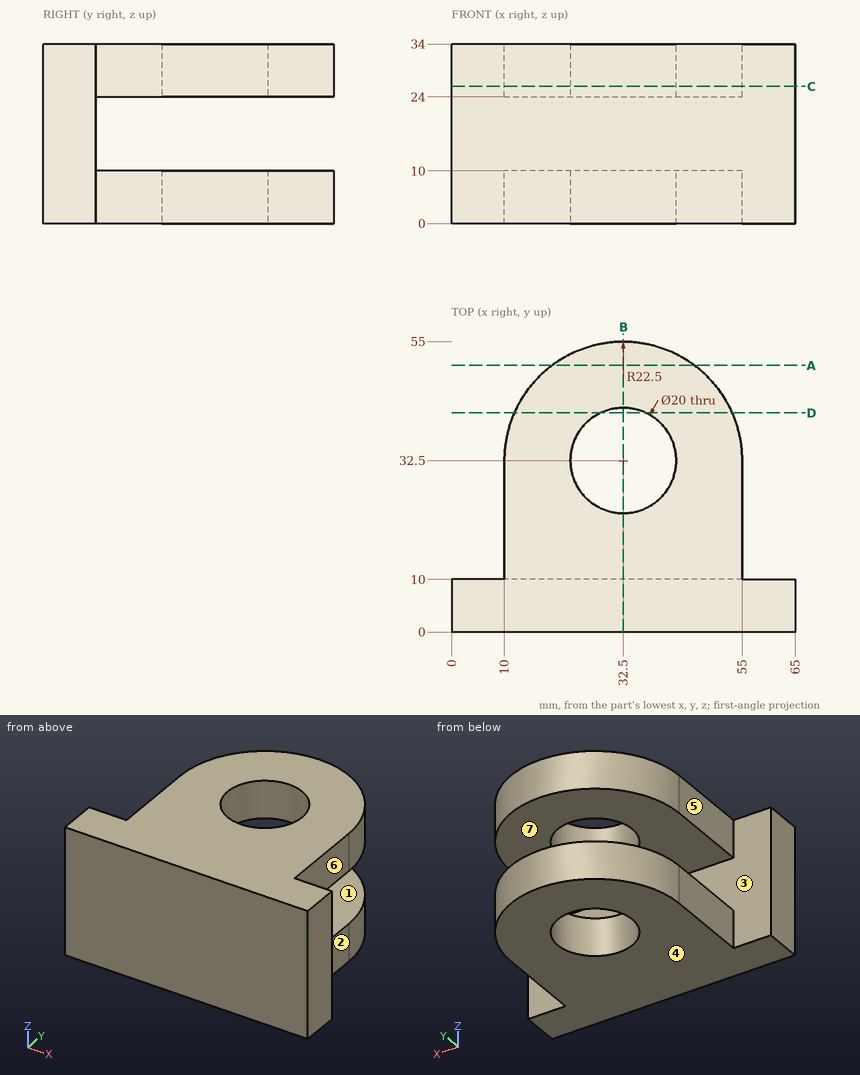
Job drawing, mm, ordinate dimensions from the low corner. One solid piece. A direction names the side the tool comes from. Coordinates: 2 decimals unless noted, no trailing zeros. Order: outer loops, then holes, each group sorted by start corner. A loop starts at its lowest first (then second) coordinate and runs counter-clockwise, first axis right, second up. Notation, with made-up numbers: M 36.5,89.5 L 80.5,89.5 A15 ccw 80.5,99.5 Z; hole C 36.25,10 d2. An arc over 180 degrees is marked long. Answer as CSV lines item,"result".
(1) Band-saw the part on B-B, the plane x = 32.5. List the corners of the cut face in (y, z).
Geometry says:
outline,"M 0,0 L 22.5,0 L 22.5,10 L 10,10 L 10,24 L 22.5,24 L 22.5,34 L 0,34 Z; M 42.5,0 L 55,0 L 55,10 L 42.5,10 Z; M 42.5,24 L 55,24 L 55,34 L 42.5,34 Z"
(2) 3-axis set-ups, long thin cutter, end or side, ignore diameter. For the marked faces 5, 6 and 7: which of +Z, -Z, +X, -X, +Y, -Y reach the whole face in a straight line?
Geometry says:
face 5,"+Z, -Z, -X, +Y"
face 6,"+Z, -Z, +X, +Y"
face 7,"+X, -X, +Y"
(3) Band-saw the part on C-C, the plane z = 26. List the corners of the cut face in (x, y).
Geometry says:
outline,"M 0,0 L 65,0 L 65,10 L 55,10 L 55,32.5 A22.5 ccw 10,32.5 L 10,10 L 0,10 Z; hole C 32.5,32.5 d20"
(4) Flat gauge pins, fed straight in: pin 1 (2 mm diameter, centred on y = 18.5, z = 12, fed in from +X); pin 2 (4 mm diameter, centred on x = 54, z = 27, fed in from -Y); pin 3 (12 mm diameter, centred on y = 39, z = 10.5, fed in from +X); pin 4 (5 mm diameter, centred on x = 50.5, z = 10.5, fed in from +Y). Where does each tip first touch, or does it go through?
Geometry says:
pin 1,"passes through"
pin 2,"stops at y = 0"
pin 3,"stops at x = 54.99"
pin 4,"stops at y = 48.76"
(5) Wall check: line 1 along Z through (x, y) = (51, 11); line 2 along X through (y, z) = (32.5, 4.5); line 3 along Y through (x, z) = (32.5, 4.5). Give the ranges that are in metal, low to high.
Geometry says:
line 1,"z = 0 to 10, 24 to 34"
line 2,"x = 10 to 22.5, 42.5 to 55"
line 3,"y = 0 to 22.5, 42.5 to 55"
(6) Band-saw the part on A-A, the plane y = 50.5. List the corners of the cut face in (x, z), then the cut area to 3 significant figures.
Geometry says:
outline,"M 19,0 L 46,0 L 46,10 L 19,10 Z; M 19,24 L 46,24 L 46,34 L 19,34 Z"
area,"540 mm2"
(7) Pull direction Z, two halves, no side cores. Call the marked faces 1, 2, 3 and 4: +Z half, -Z half, draft (parallel to the pull), parting line (faces both ways), or undercut.
Geometry says:
face 1,"undercut"
face 2,"draft"
face 3,"undercut"
face 4,"-Z half"
(8) Band-saw the part on D-D, the plane y = 41.5. List the corners of the cut face in (x, z), then the cut area to 3 significant figures.
Geometry says:
outline,"M 11.88,0 L 28.14,0 L 28.14,10 L 11.88,10 Z; M 11.88,24 L 28.14,24 L 28.14,34 L 11.88,34 Z; M 36.86,0 L 53.12,0 L 53.12,10 L 36.86,10 Z; M 36.86,24 L 53.12,24 L 53.12,34 L 36.86,34 Z"
area,"651 mm2"
